```python
from build123d import *

# Parameters (mm, degrees)
SKETCH_3_R      = 1.8
SKETCH_3_W      = 0.8
SKETCH_3_H      = 1.5
SKETCH_3_W_2    = 1
EXTRUDE_2_DEPTH = 3


with BuildPart() as part:
    # 草图3 → 凸台-拉伸2 (new body)
    with BuildSketch(Plane(origin=(0, 0, 0), x_dir=(1, 0, 0), z_dir=(0, 1, 0))):
        with BuildLine():
            Line((8.65, -27), (8.65, -21.5))
            Line((8.65, -21.5), (8.65, -20))
            Line((8.65, -20), (1.9, -20))
            Line((1.9, -20), (-0.163508327, -20))
            ThreePointArc((-0.163508327, -20), (-2.1, -20.5), (-4.036491673, -20))
            Line((-4.036491673, -20), (-20, -20))
            Line((-20, -20), (-20, -5.443559577))
            ThreePointArc((-20, -5.443559577), (-20.4, -3.7), (-20, -1.956440423))
            Line((-20, -1.956440423), (-20, 6.361726266))
            ThreePointArc((-20, 6.361726266), (-23.3, 10.3), (-20, 14.238273734))
            Line((-20, 14.238273734), (-20, 20))
            Line((-20, 20), (-16.7, 20))
            Line((-16.7, 20), (-16.7, 27))
            Line((-16.7, 27), (-27, 27))
            Line((-27, 27), (-27, -27))
            Line((-27, -27), (8.65, -27))
        make_face()
        with Locations((-23.5, -23.5)):
            Circle(SKETCH_3_R, mode=Mode.SUBTRACT)
        with Locations((-23.5, 23.5)):
            Circle(SKETCH_3_R, mode=Mode.SUBTRACT)
        Polygon((20, -18), (20, -20), (20.65, -20), (20.65, -21.5), (20.65, -27), (27, -27), (27, 27), (-4.1, 27), (-4.1, 20), (20, 20), align=None)
        with Locations((23.5, -23.5)):
            Circle(SKETCH_3_R, mode=Mode.SUBTRACT)
        with Locations((23.5, 23.5)):
            Circle(SKETCH_3_R, mode=Mode.SUBTRACT)
        Polygon((12.4, -20), (12.4, -19.5), (12.4, -18), (1.9, -18), (1.9, -20), (8.65, -20), align=None)
        Polygon((20, -20), (16.9, -20), (16.9, -19.5), (16.1, -19.5), (13.4, -19.5), (12.4, -19.5), (12.4, -20), (8.65, -20), (8.65, -21.5), (20.65, -21.5), (20.65, -20), align=None)
        Polygon((16.9, -19.5), (16.9, -20), (20, -20), (20, -18), (16.9, -18), align=None)
        with Locations((16.5, -18.75)):
            Rectangle(SKETCH_3_W, SKETCH_3_H)
        with Locations((12.9, -18.75)):
            Rectangle(SKETCH_3_W_2, SKETCH_3_H)
    extrude(amount=EXTRUDE_2_DEPTH)


solid = part.part
```
Build history of the part. All positions in model axes, mm. A direction names the side the tool comes from. Coordinates: 2 decimals unless noted, no trailing zeros. Order: outer loops, then holes, each group sorted by start corner. A loop starts at its lowest first (then second) coordinate and runs counter-clockwise, first axis right, second up.
Item 1: Tool access for faces 5 (the flat face through (-27, 1, 0)), 6 (the flat face through (16.1, 1, 19)), 7 (the flat face through (27, 1, 0)), 8 (the flat face through (-16.7, 1, -23)), 9 (the flat face through (8.65, 1, 24)): list every direction of +Z, -Z, +X, -X, +Y, -Y with a clear straight run to the whole face (end or side of a thin tool).
Filled in:
face 5: +Z, -Z, -X, +Y, -Y
face 6: +Y, -Y
face 7: +Z, -Z, +X, +Y, -Y
face 8: -Z, +Y, -Y
face 9: +Z, +Y, -Y
Item 2: Saw through at B-B on z = -23.5. List the corners of the cut face in (x, y), then the cut area to 3 significant figures.
Filled in:
outline: (-27, 0) - (-25.3, 0) - (-25.3, 3) - (-27, 3) - close; (-21.7, 0) - (-16.7, 0) - (-16.7, 3) - (-21.7, 3) - close; (-4.1, 0) - (21.7, 0) - (21.7, 3) - (-4.1, 3) - close; (25.3, 0) - (27, 0) - (27, 3) - (25.3, 3) - close
area: 103 mm2
Item 3: Saw through at C-C on y = 1.25. State how many separate pieces and enclosed holes the cut face has, then the cut area to 3 significant figures.
Filled in:
separate pieces: 1
enclosed holes: 4
area: 1,130 mm2
Item 4: Saw through at A-A on x = 23.5. List the corners of the cut face in (y, z).
Filled in:
outline: (0, -27) - (3, -27) - (3, -25.3) - (0, -25.3) - close; (0, -21.7) - (3, -21.7) - (3, 21.7) - (0, 21.7) - close; (0, 25.3) - (3, 25.3) - (3, 27) - (0, 27) - close
Item 5: Mould opens along Z. For faces 1 (the flat face through (20.65, 1, 24)), 2 (the cylindrical face through (24.468, 1.479, -25.018)), 3 (the flat face through (24, 1, 27)), 4 (the flat face through (12, 1, -27)) say: released by +Z, released by -Z, zero draft, split by the parting line, or undercut.
Filled in:
face 1: zero draft
face 2: undercut
face 3: released by +Z
face 4: released by -Z
Item 6: Saw through at D-D on z = -16. List the corners of the cut face in (x, y), then the cut area to 3 significant figures.
Filled in:
outline: (-27, 0) - (-20, 0) - (-20, 3) - (-27, 3) - close; (20, 0) - (27, 0) - (27, 3) - (20, 3) - close
area: 42.0 mm2
Item 7: Drill centre lines: L1, parallel to X at y = 1.6, z = -23.5; L2, parallel to Z at x = -23.5, y = 1.55; L3, parallel to X at y = 1.75, z = 23.5. Where is each one in solid material? Low to high.
Filled in:
L1: x = -27 to -25.3, -21.7 to -16.7, -4.1 to 21.7, 25.3 to 27
L2: z = -27 to -25.3, -21.7 to 21.7, 25.3 to 27
L3: x = -27 to -25.3, -21.7 to 8.65, 20.65 to 21.7, 25.3 to 27
